Could you check a few things on this model? Use its own coordinates, in mm. A direction names the side the tool comes from. Give positions to 0.01 mm unless a question says otherwise; leave off trailing zeros. Loops run counter-clockwise (first coordinate to the right, second up) from the corner with the lowest first, then second, coordinate; pieces in that order, holes last.
1. Thinking about a two-plate mould opening in X: for faces 3 (the cylindrical face through (-15, 0, 25)), 4 (the flat face through (12, 19, 31.401)), 5 (the conical face through (-22.12, -6.96, 30.96)), which applies, +X half, -X half, draft (parallel to the pull), parting line (faces both ways), or undercut?
2. I need wall thicknesses on line 1 along Z through (x, y) = (7, 4); line 2 along Y through (x, z) = (-14, 26.5); line 3 along X through (y, z) = (0, 30.65). Which ranges of each line are inside material? Lowest first, please.
3. Imagine slicing it at C-C (z = 27.5). List the corners of the cut face in (x, y) for me, plus the area to 3 significant figures.
4. For faces 1 (the cylindrical face through (20.633, 15.821, 22.88)), 2 (the cylindrical face through (4.769, 21.477, 30.662)), which set-ups out of +Z, -Z, +X, -X, +Y, -Y let a thin tool reach every point of the face, with its end or its side?
5. For P1, Ø1, axis at x = 20, z = 25.5, coming from the -Y side; P2, Ø5, axis at x = -11.5, z = 26, coming from the -Y side; P3, Ø1.5, axis at x = 4.5, z = 23, coming from the -Y side, each with a flat end and sliding along its axis, tell me the tip position at first contact or that it passes through.
6. Imagine slicing it at B-B (y = 0). List the corners of the cut face in (x, z) for me.
7. Imagine slicing it at A-A (x = 0). List the corners of the cut face in (y, z) for me, plus the area to 3 significant figures.
```python
from build123d import *

# Parameters (mm, degrees)
F3_D = 2


with BuildPart() as f1:
    # F0 (on Front) → F1 (revolve)
    with BuildSketch(Plane.XZ):
        Polygon((-26, 21.401275), (-4, 21.401275), (-4, 29.401275), (-21.5, 29.401275), (-22, 29.901275), (-22, 31.401275), (-23, 31.401275), (-26, 24.401275), align=None)
    revolve(axis=Axis((0, 0, 25.401275), (0, 0, 1)))

    # F3 (through all)
    with Locations(Plane(origin=(0, 0, 21.401275), x_dir=(1, 0, 0), z_dir=(0, 0, -1))):
        with Locations((-14, 0), (14, 0)):
            Hole(F3_D / 2)


solid = f1.part
```
Derived:
1. face 3: undercut
1. face 4: draft
1. face 5: parting line
2. line 1: z = 21.4 to 29.4
2. line 2: y = -20.83 to -1, 1 to 20.83
2. line 3: x = -23.32 to -22, 22 to 23.32
3. outline: circle Ø49.34 at (0, 0); hole circle Ø2 at (-14, 0); hole circle Ø8 at (0, 0); hole circle Ø2 at (14, 0)
3. area: 1,860 mm2
4. face 1: +Z, -Z
4. face 2: +Z
5. P1: stops at y = -16.56
5. P2: stops at y = -24.17
5. P3: stops at y = -25.73
6. outline: (-26, 21.4) - (-15, 21.4) - (-15, 29.4) - (-21.5, 29.4) - (-22, 29.9) - (-22, 31.4) - (-23, 31.4) - (-26, 24.4) - close; (-13, 21.4) - (-4, 21.4) - (-4, 29.4) - (-13, 29.4) - close; (4, 21.4) - (13, 21.4) - (13, 29.4) - (4, 29.4) - close; (15, 21.4) - (26, 21.4) - (26, 24.4) - (23, 31.4) - (22, 31.4) - (22, 29.9) - (21.5, 29.4) - (15, 29.4) - close
7. outline: (-26, 21.4) - (-4, 21.4) - (-4, 29.4) - (-21.5, 29.4) - (-22, 29.9) - (-22, 31.4) - (-23, 31.4) - (-26, 24.4) - close; (4, 21.4) - (26, 21.4) - (26, 24.4) - (23, 31.4) - (22, 31.4) - (22, 29.9) - (21.5, 29.4) - (4, 29.4) - close
7. area: 347 mm2
